Geometry check sheet. Reference: the model listing, model coordinates, mm. Face numbers are marked on the shaded views. Round coordinates to 2 decimals unless told otherwise and drop trailing zeros. Order: outer loops, then holes, each group sorted by start corner. A loop starts at its lowest first (then second) coordinate and runs counter-clockwise, first axis right, second up. Notation, with made-up numbers: (-18, -24.75) - (41, -24.75) arc R11 cw to (41, -6.75) - close; hole circle Ø3 at (-1, 81). An arc over 180 degrees is marked (long way). Return JSON: item names as keys, results as strings. Group by question number.
Q1. Sectioned sample at D-D, the plane x = -8.5. Record the cut outline in (y, z), then the cut area to 3 significant figures.
Q2. Draft check along Z on the marked faces 1, 2 and 3. Enter one of: pulls with the +Z half, pulls with the -Z half, needs draft (parallel to the pull), parting line crosses it, or undercut.
Q3. Sectioned sample at B-B, the plane x = 0. Record the cut outline in (y, z), then the cut area to 3 significant figures.
Q4. Sectioned sample at A-A, the plane y = 2.7. Record the cut outline in (x, z), then the cut area to 3 significant figures.
Q5. Gauge pin test, flat ends, axial feed: pin 1 Ø1.5 at (y, z) = (4, -8.5) entering from -X; pin 2 Ø1 at (x, y) = (-5.5, 3.5) entering from -Z; pin 3 Ø2 at (x, y) = (-8, 3) entering from -Z. Record the tip position at first contact, or that the pin passes through.
Q6. Material ranges on line 1 along X through (y, z) = (3.05, 0); line 2 along X through (y, z) = (4.25, -0.5); line 3 along Z through (x, y) = (-3.75, 1.75), recorded low to high.
Q7. Sectioned sample at C-C, the plane z = 9.5. Record the cut outline in (x, y), then the cut area to 3 significant figures.
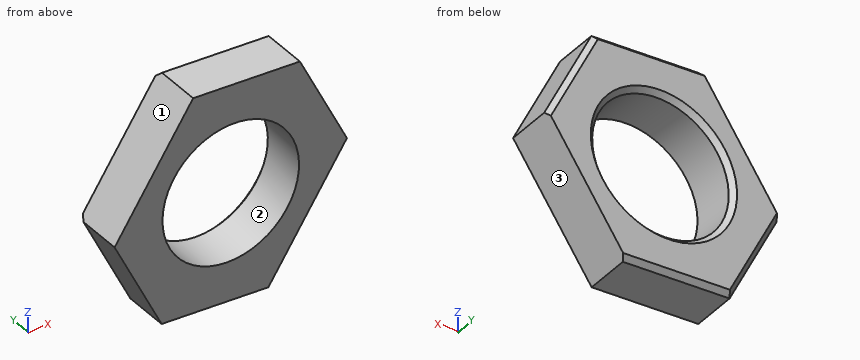
```python
from build123d import *

# Parameters (mm, degrees)
SKETCH1_R           = 7
BOSS_EXTRUDE1_DEPTH = 5
CHAMFER1_SIZE       = 0.5
CUT_EXTRUDE1_DEPTH  = 18.76901793


with BuildPart() as part:
    # Sketch1 → Boss-Extrude1 (new body)
    with BuildSketch(Plane(origin=(0, 0, 0), x_dir=(1, 0, 0), z_dir=(0, 1, 0))):
        Polygon((7.08862867, -10.539671575), (12.671937667, 0.869096719), (5.583308997, 11.408768294), (-7.08862867, 10.539671575), (-12.671937667, -0.869096719), (-5.583308997, -11.408768294), align=None)
        with Locations(Location((0, 0, 0), (0, 0, 270))):
            Circle(SKETCH1_R, mode=Mode.SUBTRACT)
    extrude(amount=BOSS_EXTRUDE1_DEPTH)

    # Chamfer1
    chamfer1_edges = [part.edges().sort_by_distance(p)[0] for p in [
        (9.127623332, 5, -6.138932506),
        (-0.752659837, 5, -10.974219934),
        (-9.880283168, 5, -4.835287428),
        (0, 5, -7),
        (-9.127623332, 5, 6.138932506),
        (0.752659837, 5, 10.974219934),
        (9.880283168, 5, 4.835287428),
    ]]
    chamfer(chamfer1_edges, length=CHAMFER1_SIZE)

    # Sketch2 → Cut-Extrude1 (cut, through all)
    with BuildSketch(Plane(origin=(0, 5, 0), x_dir=(1, 0, 0), z_dir=(0, 1, 0))):
        Polygon((-12.369841003, 1.369496951), (-3.313446114, -12.095932292), (-6.221668225, -14.051904686), (-15.278063114, -0.586475443), align=None)
        Polygon((3.396053842, 11.973107643), (6.304275954, 13.929080037), (15.360670843, 0.463650794), (12.452448732, -1.4923216), align=None)
    extrude(amount=-CUT_EXTRUDE1_DEPTH, mode=Mode.SUBTRACT)


solid = part.part
```
Reply:
{
 "1": {"outline": "(0, -7.66) - (4.5, -7.66) - (5, -6.52) - (5, 4.38) - (0, 4.38) - close", "area": "59.9 mm^2"},
 "2": {"face 1": "pulls with the +Z half", "face 2": "undercut", "face 3": "pulls with the -Z half"},
 "3": {"outline": "(0, -11.03) - (4.5, -11.03) - (5, -10.52) - (5, -7.5) - (4.5, -7) - (0, -7) - close; (0, 7) - (4.5, 7) - (5, 7.5) - (5, 10.52) - (4.5, 11.03) - (0, 11.03) - close", "area": "39.8 mm^2"},
 "4": {"outline": "(-11.91, -0.69) - (-7.09, -10.54) - (3.86, -11.29) - (11.91, 0.69) - (7.09, 10.54) - (-3.86, 11.29) - close; hole circle Ø14 at (0, 0)", "area": "225 mm^2"},
 "5": {"pin 1": "x = -8.45", "pin 2": "z = -10.68", "pin 3": "z = -10.55"},
 "6": {"line 1": "-11.45 to -7, 7 to 11.45", "line 2": "-11.79 to -6.98, 6.98 to 11.11", "line 3": "-10.77 to -5.91, 5.91 to 11.28"},
 "7": {"outline": "(-5.06, 0) - (7.6, 0) - (7.6, 4.5) - (7.04, 5) - (-5.06, 5) - close", "area": "63.1 mm^2"}
}
